from build123d import *
from build123d.topology import SkipClean

# Parameters (mm, degrees)
SKETCH1_R              = 11.43
MAIN_SHAFT_DEPTH       = 33.3375
NEEDLE_HOLE_DEPTH      = 69.606453231
NEEDLE_HOLE_DEPTH_BACK = 69.606453231
SKETCH5_R              = 1.27
SKETCH7_R              = 10.16
SYRINGE_SLOT_DEPTH     = 40.132
SPRING_START           = -22.733
SKETCH9_R              = 10.16
SPRING_SLOT_DEPTH      = 22.733
TABS_START             = -1.27
TABS_DEPTH             = 1.27
SKETCH12_W             = 40.64
SKETCH12_H             = 22.86
SYRINGE_INSERT_DEPTH   = 43.734300331


with BuildPart() as part:
    # Sketch1 → Main Shaft (new, symmetric)
    with BuildSketch(Plane(origin=(0, 0, 0), x_dir=(0, 0, -1), z_dir=(1, 0, 0))):
        Circle(SKETCH1_R)
    extrude(amount=MAIN_SHAFT_DEPTH, both=True)

    # Sketch4 → Bumpout (revolve)
    with BuildSketch(Plane.XY):
        with BuildLine():
            Line((-33.3375, 0), (-33.3375, 6.35))
            ThreePointArc((-33.3375, 6.35), (-37.827628061, 4.490128061), (-39.6875, 0))
            Line((-39.6875, 0), (-33.3375, 0))
        make_face()
    revolve(axis=Axis((88.99, 0, 0), (-1, 0, 0)))

    # Sketch5 → Needle Hole (cut, two sides: drawn at the far end of the back side and taken through both)
    with BuildSketch(Plane.ZY.offset(33.3375).offset(-NEEDLE_HOLE_DEPTH_BACK)):
        with Locations(Location((0, 0, 0), (0, 0, 180))):
            Circle(SKETCH5_R)
    extrude(amount=NEEDLE_HOLE_DEPTH + NEEDLE_HOLE_DEPTH_BACK, mode=Mode.SUBTRACT)

    # Sketch7 → Syringe Slot (cut)
    with BuildSketch(Plane.ZY.offset(30.7975)):
        Circle(SKETCH7_R)
    extrude(amount=-SYRINGE_SLOT_DEPTH, mode=Mode.SUBTRACT)

    # Sketch9 → Spring Slot (cut)
    with BuildSketch(Plane(origin=(33.3375, 0, 0), x_dir=(0, 0, -1), z_dir=(1, 0, 0)).offset(SPRING_START)):
        with Locations(Location((0, 0, 0), (0, 0, 180))):
            Circle(SKETCH9_R)
    extrude(amount=SPRING_SLOT_DEPTH, mode=Mode.SUBTRACT)

    # Sketch11 → Tabs (cut)
    with SkipClean():  # the faces are left unmerged after this step: merging them gives an invalid solid
        with BuildSketch(Plane(origin=(10.6045, 0, 0), x_dir=(0, 0, -1), z_dir=(1, 0, 0)).offset(TABS_START)):
            with BuildLine():
                Line((-1.27, 8.798818102), (-1.451428571, 10.055792117))
                ThreePointArc((-1.451428571, 10.055792117), (-10.16, 0), (-1.451428571, -10.055792117))
                Line((-1.451428571, -10.055792117), (-1.27, -8.798818102))
                ThreePointArc((-1.27, -8.798818102), (-8.89, 0), (-1.27, 8.798818102))
            make_face()
            with BuildLine():
                Line((1.27, 8.798818102), (1.451428571, 10.055792117))
                ThreePointArc((1.451428571, 10.055792117), (10.16, 0), (1.451428571, -10.055792117))
                Line((1.451428571, -10.055792117), (1.27, -8.798818102))
                ThreePointArc((1.27, -8.798818102), (8.89, 0), (1.27, 8.798818102))
            make_face()
        extrude(amount=TABS_DEPTH, mode=Mode.SUBTRACT)

    # Sketch12 → Syringe Insert (cut, through all)
    with BuildSketch(Plane.XY):
        with Locations((-13.0175, 0)):
            Rectangle(SKETCH12_W, SKETCH12_H)
    extrude(amount=-SYRINGE_INSERT_DEPTH, mode=Mode.SUBTRACT)


solid = part.part
The model under review builds one solid part; all positions refer to its coordinate system, in mm. A direction names the side the tool comes from. Give positions to 0.01 mm unless a question says otherwise; leave off trailing zeros. Write each loop counter-clockwise with the first axis right and the second up, starting at its lowest first coordinate (ties: lowest second). Pieces come first, ordered by that corner, then holes.
1. Draft analysis for pull direction X (two halves, no side actions). For faces 1 (the cylindrical face through (9.96, -0.18, -8.89)), 2 (the flat face through (10.604, 0, 2)), 3 (the flat face through (-21, 11, 0)), state which applies: +X half, -X half, draft (parallel to the pull), parting line (faces both ways), or undercut.
2. Add section C-C, the plane x = 14.5. Write out the cut boundary in (y, z).
3. Wall thickness on L1, parallel to X at y = -3.25, z = 7.75; L2, parallel to Z at x = 9.5, y = 3.25; L3, parallel to X at y = 3.75, z = 4: over which ranges is each line inside the solid? List them lowest first.
4. Add section D-D, the plane z = -8.25. Write out the cut boundary in (x, y), plus the area to 3 significant figures.
5. Add section B-B, the plane z = 5. Write out the cut boundary in (x, y).
6. Tool access review of faces 4 (the flat face through (9.334, 0, 2)), 5 (the flat face through (7.302, -0.05, -10.34)), 6 (the cylindrical face through (9.96, -0.18, 8.89)): name each direction out of +Z, -Z, +X, -X, +Y, -Y from which nothing blocks a thin tool from reaching the whole face with its end or side.
7. For P1, Ø8, axis at y = -1, z = 4, coming from the +X side; P2, Ø12, axis at x = -21.5, y = 8, coming from the +Z side; P3, Ø5.5, axis at y = 4.5, z = -6.5, coming from the -X side; P4, Ø4, axis at y = 0, z = 0, coming from the -X side, all flat-tipped, find the tip position at first contact; note any pin that passes through.
8. Add section A-A, the plane y = 0. Write out the cut boundary in (x, z).
Worked answers:
1. face 1: draft
1. face 2: +X half
1. face 3: undercut
2. outline: circle Ø22.86 at (0, 0); hole circle Ø20.32 at (0, 0)
3. L1: x = -33.34 to -30.8, 9.33 to 10.6
3. L2: z = -10.96 to -9.63, -8.27 to 8.27, 9.63 to 10.96
3. L3: x = -36.54 to -30.8, 9.33 to 10.6
4. outline: (7.3, -7.91) - (33.34, -7.91) - (33.34, -5.93) - (7.3, -5.93) - close; (7.3, 5.93) - (33.34, 5.93) - (33.34, 7.91) - (7.3, 7.91) - close; (9.33, -3.31) - (10.6, -3.31) - (10.6, 3.31) - (9.33, 3.31) - close
4. area: 112 mm2
5. outline: (-33.34, -10.28) - (33.34, -10.28) - (33.34, -8.84) - (-30.8, -8.84) - (-30.8, 8.84) - (33.34, 8.84) - (33.34, 10.28) - (-33.34, 10.28) - (-33.34, 3.91) arc R3.91 ccw to (-33.34, -3.91) - close; (9.33, -7.35) - (10.6, -7.35) - (10.6, 7.35) - (9.33, 7.35) - close
6. face 4: none
6. face 5: -Z, -X, +Y, -Y
6. face 6: +X
7. P1: stops at x = 10.6
7. P2: stops at z = 11.25
7. P3: stops at x = -37.04
7. P4: stops at x = -39.56
8. outline: (-39.56, -1.27) arc R6.35 ccw to (-33.34, -6.35) - (-33.34, -1.27) - close; (-39.56, 1.27) - (-30.8, 1.27) - (-30.8, 10.16) - (33.34, 10.16) - (33.34, 11.43) - (-33.34, 11.43) - (-33.34, 6.35) arc R6.35 ccw to start; (7.3, -11.43) - (33.34, -11.43) - (33.34, -10.16) - (7.3, -10.16) - close; (9.33, -8.89) - (10.6, -8.89) - (10.6, -1.27) - (9.33, -1.27) - close; (9.33, 1.27) - (10.6, 1.27) - (10.6, 8.89) - (9.33, 8.89) - close
